Can you work these out from the drawing? Everything is in mm from the part's minimum corner. A direction names the side the tool comes from. Round coordinates to 2 decimals unless told otherwise and drop trailing zeros. Write each loop counter-clockwise with the first axis right and the second up, starting at its lowest first coordinate (ties: lowest second). Pieces come first, ordered by that corner, then holes. Notation, with made-up numbers: (72.25, 7) -> (100.25, 7) arc R13 cw to (100.25, 11) -> close; hole circle Ø6 at (-30, -32). An arc over 180 degrees is marked (long way). One line per question, with ' | ' between items. Start each with the question number.
1. For pin 1 Ø3 at (x, z) = (22, 13) entering from +Y; pin 2 Ø3.5 at (x, z) = (11, 10) entering from +Y, each with a flat end and sliding along its axis, tell me the tip position at first contact or that it passes through.
2. For the marked faces 1, 2 and 3, which set-ups out of +Z, -Z, +X, -X, +Y, -Y let a thin tool reach every point of the face, with its end or its side?
3. Imagine slicing it at B-B, the plane y = 4. List the corners of the cut face in (x, z) for me, and give its area (3 significant figures).
4. Imagine slicing it at A-A, the plane x = 22. List the corners of the cut face in (y, z) for me.
5. Imagine slicing it at D-D, the plane x = 18.25. List the corners of the cut face in (y, z) for me.
6. Thinking about a two-plate mould opening in Z: for the marked faces 4, 5, 6 and 7, which applies, released by +Z, released by -Z, zero draft, split by the parting line, or undercut?
7. If I drill on line 1 along X through (y, z) = (3.1, 3); line 2 along X through (y, z) = (2.3, 13); line 3 along Z through (x, y) = (6.5, 5.55), over which ranges is the centre line in solid material (lowest first)? Write a range as [from, to].
8. Imagine slicing it at C-C, the plane z = 11.5. List the corners of the cut face in (x, y) for me.
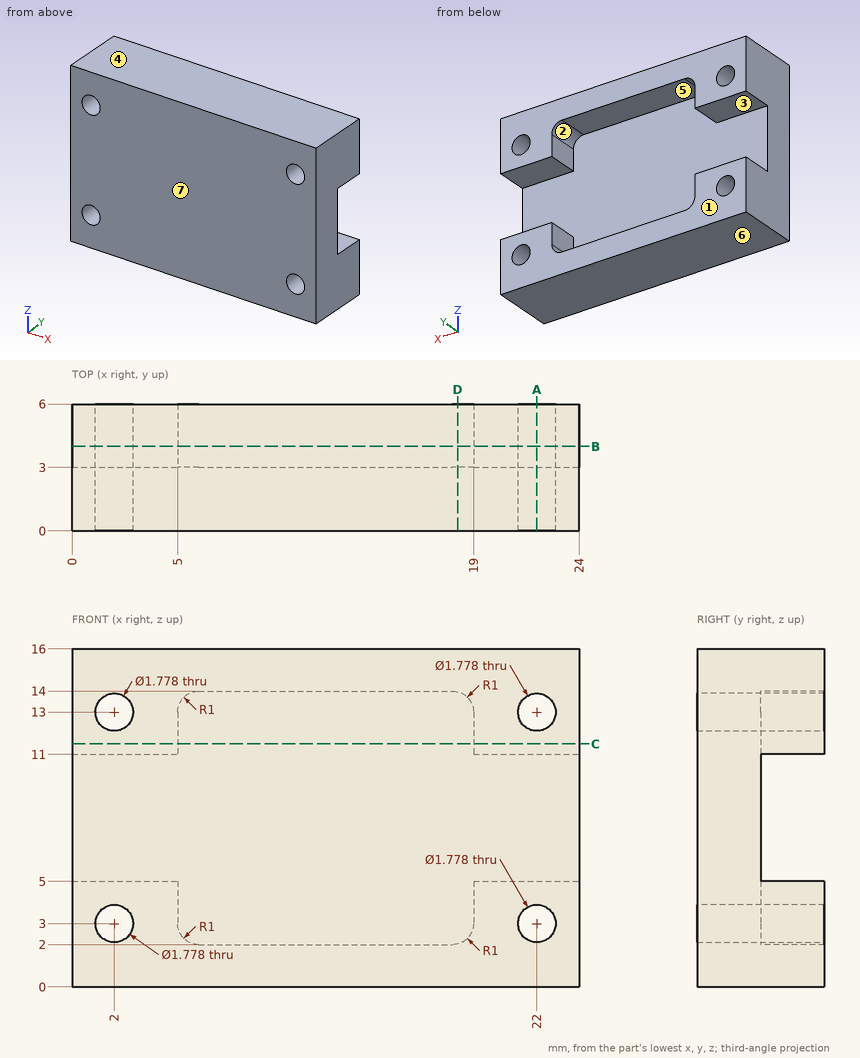
Geometry results:
1) pin 1: stops at y = 6 | pin 2: stops at y = 3
2) face 1: +Z, -Z, +X, -X, +Y | face 2: +Y | face 3: +X, -X, +Y
3) outline: (0, 0) -> (24, 0) -> (24, 5) -> (19, 5) -> (19, 3) arc R1 cw to (18, 2) -> (6, 2) arc R1 cw to (5, 3) -> (5, 5) -> (0, 5) -> close; (0, 11) -> (5, 11) -> (5, 13) arc R1 cw to (6, 14) -> (18, 14) arc R1 cw to (19, 13) -> (19, 11) -> (24, 11) -> (24, 16) -> (0, 16) -> close; hole circle Ø1.78 at (2, 3); hole circle Ø1.78 at (2, 13); hole circle Ø1.78 at (22, 3); hole circle Ø1.78 at (22, 13) | area: 147 mm2
4) outline: (0, 0) -> (6, 0) -> (6, 2.11) -> (0, 2.11) -> close; (0, 3.89) -> (6, 3.89) -> (6, 5) -> (3, 5) -> (3, 11) -> (6, 11) -> (6, 12.11) -> (0, 12.11) -> close; (0, 13.89) -> (6, 13.89) -> (6, 16) -> (0, 16) -> close
5) outline: (0, 0) -> (6, 0) -> (6, 2.03) -> (3, 2.03) -> (3, 13.97) -> (6, 13.97) -> (6, 16) -> (0, 16) -> close
6) face 4: released by +Z | face 5: undercut | face 6: released by -Z | face 7: zero draft
7) line 1: x = [0, 1.11], [2.89, 5], [19, 21.11], [22.89, 24] | line 2: x = [0, 1.11], [2.89, 21.11], [22.89, 24] | line 3: z = [0, 2], [14, 16]
8) outline: (0, 0) -> (24, 0) -> (24, 6) -> (19, 6) -> (19, 3) -> (5, 3) -> (5, 6) -> (0, 6) -> close
